from build123d import *

# Parameters (mm, degrees)
SKETCH1_W            = 30
SKETCH1_H            = 55
BOSS_EXTRUDE1_DEPTH  = 1.5
SKETCH2_W            = 8
SKETCH2_H            = 15
CUT_EXTRUDE1_DEPTH   = 43.238610108
SKETCH3_W            = 7
SKETCH3_H            = 3
BOSS_EXTRUDE2_DEPTH  = 8
SKETCH6_W            = 3
SKETCH6_H            = 8
BOSS_EXTRUDE3_DEPTH  = 3
M4_CLEARANCE_HOLE1_D = 4.5
FILLET1_R            = 2


with BuildPart() as part:
    # Sketch1 → Boss-Extrude1 (new, symmetric)
    with BuildSketch(Plane.XY):
        with Locations((0.944117647, -11.498529412)):
            Rectangle(SKETCH1_W, SKETCH1_H)
    extrude(amount=BOSS_EXTRUDE1_DEPTH, both=True)

    # Sketch2 → Cut-Extrude1 (cut, through all)
    with BuildSketch(Plane.XY.offset(1.5)):
        with Locations((11.944117647, 8.501470588)):
            Rectangle(SKETCH2_W, SKETCH2_H)
    extrude(amount=-CUT_EXTRUDE1_DEPTH, mode=Mode.SUBTRACT)

    # Sketch3 → Boss-Extrude2 (add)
    with BuildSketch(Plane(origin=(0, -38.998529412, 0), x_dir=(-1, 0, 0), z_dir=(0, -1, 0))):
        with Locations((-12.444117647, 0)):
            Rectangle(SKETCH3_W, SKETCH3_H)
    extrude(amount=BOSS_EXTRUDE2_DEPTH)

    # Sketch6 → Boss-Extrude3 (add)
    with BuildSketch(Plane(origin=(15.944117647, 0, 0), x_dir=(0, 0, -1), z_dir=(1, 0, 0))):
        with Locations((0, -42.998529412)):
            Rectangle(SKETCH6_W, SKETCH6_H)
    extrude(amount=BOSS_EXTRUDE3_DEPTH)

    # M4 Clearance Hole1 (through all)
    with Locations(Plane.XY.offset(1.5)):
        with Locations((-7.805882353, 11.001470588), (13.944117647, -42.998529412)):
            Hole(M4_CLEARANCE_HOLE1_D / 2)

    # Fillet1
    fillet1_edges = [part.edges().sort_by_distance(p)[0] for p in [
        (7.944117647, 16.001470588, 0),
        (15.944117647, 1.001470588, 0),
        (18.944117647, -46.998529412, 0),
        (18.944117647, -38.998529412, 0),
        (-14.055882353, 16.001470588, 0),
        (-14.055882353, -38.998529412, 0),
    ]]
    fillet(fillet1_edges, radius=FILLET1_R)


solid = part.part
The model under review builds one solid part; all positions refer to its coordinate system, in mm. A direction names the side the tool comes from. Give positions to 0.01 mm unless a question says otherwise; leave off trailing zeros. Loops run counter-clockwise (first coordinate to the right, second up) from the corner with the lowest first, then second, coordinate; pieces in that order, holes last. Notation, with made-up numbers: (7.25, -6.5) -> (13.25, -6.5) arc R12 ccw to (13.25, 3.5) -> close; hole circle Ø9 at (42.5, 48). An arc over 180 degrees is marked (long way). Answer as a JSON object with one key per item and string values. Group by question number.
Q1. Draft analysis for pull direction Y (two halves, no side actions). For faces 4 (the cylindrical face through (-6.148, 12.522, -0.021)), 5 (the flat face through (-14.056, -12, 0)), 6 (the cylindrical face through (7.374, 15.4, -0.021)), 7 (the cylindrical face through (12.906, -44.995, -0.021)), state which applies: pulls with the +Y half, pulls with the -Y half, needs draft (parallel to the pull), parting line crosses it, or undercut.
Q2. Wall thickness on line 1 along X through (y, z) = (-26, 0.55); line 2 along Y through (x, z) = (5, 1.35); line 3 along Y through (x, z) = (11.5, 1.2): over which ranges is each line inside the solid? List them lowest first.
Q3. Insertion check: pin 1 (1.5 mm diameter, centred on y = -6, z = 0, fed in from +X); pin 2 (1.5 mm diameter, centred on y = -40.5, z = 0.5, fed in from +X). Each pin has a flat end and moves straight along its axis. Give the tip position at first contact, or say it passes through.
Q4. Take a section at A-A (x = -7.5). Write out the cut boundary in (y, z).
Q5. Take a section at D-D (x = -4). Write out the cut boundary in (y, z), plus the area to 3 significant figures.
Q6. Take a section at B-B (z = -0.05). Write out the cut boundary in (x, y), plus the area to 3 significant figures.
Q7. Take a section at C-C (y = 5.5). Write out the cut boundary in (x, z).
Q8. Tool access review of faces 1 (the flat face through (11, 1.001, 0)), 2 (the flat face through (8.944, -43, 0)), 3 (the flat face through (-1, -16, 1.5)): name each direction out of +Z, -Z, +X, -X, +Y, -Y from which nothing blocks a thin tool from reaching the whole face with its end or side.
Answer below:
{
 "1": {"face 4": "undercut", "face 5": "needs draft", "face 6": "pulls with the +Y half", "face 7": "undercut"},
 "2": {"line 1": "x = -14.06 to 15.94", "line 2": "y = -39 to 16", "line 3": "y = -47 to 1"},
 "3": {"pin 1": "stops at x = 15.94", "pin 2": "stops at x = 18.94"},
 "4": {"outline": "(-39, -1.5) -> (8.77, -1.5) -> (8.77, 1.5) -> (-39, 1.5) -> close; (13.23, -1.5) -> (16, -1.5) -> (16, 1.5) -> (13.23, 1.5) -> close"},
 "5": {"outline": "(-39, -1.5) -> (16, -1.5) -> (16, 1.5) -> (-39, 1.5) -> close", "area": "165 mm2"},
 "6": {"outline": "(-14.06, -37) arc R2 ccw to (-12.06, -39) -> (8.94, -39) -> (8.94, -47) -> (16.94, -47) arc R2 ccw to (18.94, -45) -> (18.94, -41) arc R2 ccw to (16.94, -39) -> (15.94, -39) -> (15.94, -1) arc R2 ccw to (13.94, 1) -> (7.94, 1) -> (7.94, 14) arc R2 ccw to (5.94, 16) -> (-12.06, 16) arc R2 ccw to (-14.06, 14) -> close; hole circle Ø4.5 at (-7.81, 11); hole circle Ø4.5 at (13.94, -43)", "area": "1,570 mm2"},
 "7": {"outline": "(-14.06, -1.5) -> (7.94, -1.5) -> (7.94, 1.5) -> (-14.06, 1.5) -> close"},
 "8": {"face 1": "+Z, -Z, +X, +Y", "face 2": "+Z, -Z, -X, -Y", "face 3": "+Z, +X, -X, +Y, -Y"}
}
